```python
from build123d import *

# Parameters (mm, degrees)
SKETCH_2_W             = 34
SKETCH_2_H             = 24
EXTRUDE_1_DEPTH        = 1
CUT_EXTRUDE_2_DEPTH    = 1
SKETCH_4_W             = 2
SKETCH_4_H             = 0.5
CUT_EXTRUDE_3_DEPTH    = 3
SKETCH_5_W             = 1.5
SKETCH_5_H             = 0.5
CUT_EXTRUDE_4_DEPTH    = 3
SKETCH_6_W             = 0.2
SKETCH_6_H             = 0.5
CUT_EXTRUDE_6_DEPTH    = 1.2
SKETCH_7_W             = 0.2
SKETCH_7_H             = 0.5
CUT_EXTRUDE_7_DEPTH    = 1
PATTERN_LINEAR_1_COUNT = 2
PATTERN_LINEAR_1_PITCH = 2.917


with BuildPart() as part:
    # 草图2 → 凸台-拉伸1 (new body)
    with BuildSketch(Plane(origin=(0, 0, 0), x_dir=(1, 0, 0), z_dir=(0, 1, 0))):
        Rectangle(SKETCH_2_W, SKETCH_2_H)
    extrude(amount=EXTRUDE_1_DEPTH)

    # 草图3 → 切除-拉伸2 (cut)
    with BuildSketch(Plane(origin=(0, 1, 0), x_dir=(1, 0, 0), z_dir=(0, 1, 0))):
        with BuildLine():
            Line((2.852693105, 6.5), (0, 6.5))
            Line((0, 6.5), (0, -6.5))
            add(Edge.make_bspline(
                [(4, -3.960322269), (3.291830105, -5.33321398), (1.554438327, -6.399660403), (0, -6.5)],
                knots=[0.726831855, 0.726831855, 0.726831855, 0.726831855, 0.974825143, 0.974825143, 0.974825143, 0.974825143], degree=3))
            Line((4, -3.960322269), (4, 0))
            add(Edge.make_bspline(
                [(4, 2.711962076), (3.993732983, 1.774234816), (3.903899915, 0.904091061), (4, 0)],
                knots=[0.362705738, 0.362705738, 0.362705738, 0.362705738, 0.509475385, 0.509475385, 0.509475385, 0.509475385], degree=3))
            Line((4, 2.711962076), (4, 2.909239089))
            add(Edge.make_bspline(
                [(2.852693105, 6.5), (3.766558676, 5.806047297), (3.99030544, 4.279578326), (4, 2.909239089)],
                knots=[0.140232201, 0.140232201, 0.140232201, 0.140232201, 0.352466659, 0.352466659, 0.352466659, 0.352466659], degree=3))
        make_face()
        with BuildLine():
            Line((0, -6.5), (0, 6.5))
            Line((0, 6.5), (-2.852693105, 6.5))
            add(Edge.make_bspline(
                [(-2.852693105, 6.5), (-3.766558676, 5.806047297), (-3.99030544, 4.279578326), (-4, 2.909239089)],
                knots=[0.140232201, 0.140232201, 0.140232201, 0.140232201, 0.352466659, 0.352466659, 0.352466659, 0.352466659], degree=3))
            Line((-4, 2.909239089), (-4, 2.711962076))
            add(Edge.make_bspline(
                [(-4, 2.711962076), (-3.993732983, 1.774234816), (-3.903899915, 0.904091061), (-4, 0)],
                knots=[0.362705738, 0.362705738, 0.362705738, 0.362705738, 0.509475385, 0.509475385, 0.509475385, 0.509475385], degree=3))
            Line((-4, 0), (-4, -3.960322269))
            add(Edge.make_bspline(
                [(-4, -3.960322269), (-3.291830105, -5.33321398), (-1.554438327, -6.399660403), (0, -6.5)],
                knots=[0.726831855, 0.726831855, 0.726831855, 0.726831855, 0.974825143, 0.974825143, 0.974825143, 0.974825143], degree=3))
        make_face()
        with BuildLine():
            add(Edge.make_bspline(
                [(0, 6.5), (0.096578276, 6.539787769), (0.190890779, 6.57622482), (0.282988495, 6.609417035)],
                knots=[0, 0, 0, 0, 0.010078853, 0.010078853, 0.010078853, 0.010078853], degree=3))
            Line((0, 6.5), (2.852693105, 6.5))
            add(Edge.make_bspline(
                [(0.282988495, 6.609417035), (1.47229303, 7.038044945), (2.292262606, 6.925568347), (2.852693105, 6.5)],
                knots=[0.010078853, 0.010078853, 0.010078853, 0.010078853, 0.140232201, 0.140232201, 0.140232201, 0.140232201], degree=3))
        make_face()
        with BuildLine():
            Line((-2.852693105, 6.5), (0, 6.5))
            add(Edge.make_bspline(
                [(0, 6.5), (-0.094670577, 6.539001846), (-0.187164009, 6.574784039), (-0.277528318, 6.60744631)],
                knots=[0, 0, 0, 0, 0.009879767, 0.009879767, 0.009879767, 0.009879767], degree=3))
            add(Edge.make_bspline(
                [(-0.277528318, 6.60744631), (-1.469783924, 7.038388308), (-2.291405355, 6.926219308), (-2.852693105, 6.5)],
                knots=[0.009879767, 0.009879767, 0.009879767, 0.009879767, 0.140232201, 0.140232201, 0.140232201, 0.140232201], degree=3))
        make_face()
        with BuildLine():
            add(Edge.make_bspline(
                [(0, 6.5), (-0.094670577, 6.539001846), (-0.187164009, 6.574784039), (-0.277528318, 6.60744631)],
                knots=[0, 0, 0, 0, 0.009879767, 0.009879767, 0.009879767, 0.009879767], degree=3))
            add(Edge.make_bspline(
                [(0, 6.5), (0.096578276, 6.539787769), (0.190890779, 6.57622482), (0.282988495, 6.609417035)],
                knots=[0, 0, 0, 0, 0.010078853, 0.010078853, 0.010078853, 0.010078853], degree=3))
            add(Edge.make_bspline(
                [(0.282988495, 6.609417035), (-0.002451987, 7.75268333), (-0.277528318, 6.60744631)],
                knots=[0, 0, 0, 1, 1, 1], degree=2))
        make_face()
        with BuildLine():
            add(Edge.make_bspline(
                [(-4, 0), (-4.115462181, -1.086245927), (-4.588613513, -2.485549912), (-4.117125058, -3.733258083), (-4, -3.960322269)],
                knots=[0.509475385, 0.509475385, 0.509475385, 0.509475385, 0.685815952, 0.726831855, 0.726831855, 0.726831855, 0.726831855], degree=3))
            Line((-4, -3.960322269), (-4, 0))
        make_face()
        with BuildLine():
            Line((4, 0), (4, -3.960322269))
            add(Edge.make_bspline(
                [(4, 0), (4.115462181, -1.086245927), (4.588613513, -2.485549912), (4.117125058, -3.733258083), (4, -3.960322269)],
                knots=[0.509475385, 0.509475385, 0.509475385, 0.509475385, 0.685815952, 0.726831855, 0.726831855, 0.726831855, 0.726831855], degree=3))
        make_face()
    extrude(amount=-CUT_EXTRUDE_2_DEPTH, mode=Mode.SUBTRACT)

    # 草图4 → 切除-拉伸3 (cut)
    with BuildSketch(Plane.XY.offset(8)):
        with Locations((0, 0.5)):
            Rectangle(SKETCH_4_W, SKETCH_4_H)
    extrude(amount=-CUT_EXTRUDE_3_DEPTH, mode=Mode.SUBTRACT)

    # 草图5 → 切除-拉伸4 (cut)
    with BuildSketch(Plane(origin=(0, 0, -8), x_dir=(-1, 0, 0), z_dir=(0, 0, -1))):
        with Locations((1.458123879, 0.5)):
            Rectangle(SKETCH_5_W, SKETCH_5_H)
        with Locations((-1.458123879, 0.5)):
            Rectangle(SKETCH_5_W, SKETCH_5_H)
    extrude(amount=-CUT_EXTRUDE_4_DEPTH, mode=Mode.SUBTRACT)

    # 草图6 → 切除-拉伸6 (cut)
    with BuildSketch(Plane(origin=(0, 0, 8), x_dir=(-1, 0, 0), z_dir=(0, 0, -1))):
        with Locations((1.1, 0.5)):
            Rectangle(SKETCH_6_W, SKETCH_6_H)
        Polygon((1, 0.75), (-1, 0.25), (1, 0.25), align=None)
        Polygon((1, 0.75), (-1, 0.25), (-1, 0.75), align=None)
        with Locations((-1.1, 0.5)):
            Rectangle(SKETCH_6_W, SKETCH_6_H)
    extrude(amount=CUT_EXTRUDE_6_DEPTH, mode=Mode.SUBTRACT)

    # 草图7 → 切除-拉伸7 (cut)
    with BuildSketch(Plane.XY.offset(-8)):
        Polygon((-0.708123879, 0.25), (-2.208123879, 0.75), (-2.208123879, 0.25), align=None)
        with Locations((-2.308123879, 0.5)):
            Rectangle(SKETCH_7_W, SKETCH_7_H)
        Polygon((-0.708123879, 0.25), (-2.208123879, 0.75), (-0.708123879, 0.75), align=None)
        with Locations((-0.608123879, 0.5)):
            Rectangle(SKETCH_7_W, SKETCH_7_H)
    cut_extrude_7 = extrude(amount=CUT_EXTRUDE_7_DEPTH, mode=Mode.SUBTRACT)

    # 阵列(线性)1: 切除-拉伸7 ×2
    with Locations(*[(i * PATTERN_LINEAR_1_PITCH, 0, 0) for i in range(1, PATTERN_LINEAR_1_COUNT)]):
        add(cut_extrude_7, mode=Mode.SUBTRACT)


solid = part.part
```
For this review, take the finished solid that the model builds, in its own axes (mm). A direction names the side the tool comes from. Round coordinates to 2 decimals unless told otherwise and drop trailing zeros. Use a Markdown table: item, result.
Item 1: For line 1 along X through (y, z) = (0.6, -6.5); line 2 along X through (y, z) = (0.6, -6.25); line 3 along Z through (x, y) = (1.5, 0.45), list the stretches that pass through material, from the lowest coordinate up. Write a range as [from, to].
Resolved:
| item | result |
|---|---|
| line 1 | x = [-17, -2.85], [2.85, 17] |
| line 2 | x = [-17, -3.12], [3.12, 17] |
| line 3 | z = [-12, -8], [6.13, 12] |
Item 2: Machinability: for faces 5 (the flat face through (-1, 0.75, -7)), 6 (the flat face through (-0.2, 0.5, 12)), which of the approach directions +Z, -Z, +X, -X, +Y, -Y give a long, thin tool a straight path to every point of the face, cutting with its end or side? Answer none if there is none.
Resolved:
| item | result |
|---|---|
| face 5 | none |
| face 6 | +Z, +X, -X, +Y, -Y |
Item 3: Draft analysis for pull direction X (two halves, no side actions). For faces 1 (the flat face through (17, 0.5, 0.2)), 2 (the flat face through (-17, 0.5, 0.2)), 3 (the flat face through (1, 0.75, -7)), 4 (the flat face through (-0.2, 0.5, -12)), state which applies: +X half, -X half, draft (parallel to the pull), parting line (faces both ways), or undercut.
Resolved:
| item | result |
|---|---|
| face 1 | +X half |
| face 2 | -X half |
| face 3 | undercut |
| face 4 | draft |
